```python
from build123d import *

# Parameters (mm, degrees)
SKETCH1_W               = 266.7
SKETCH1_H               = 215.9
BASE_FLANGE1_DEPTH      = 1.5748
SKETCH6_R               = 3.96875
CUT_EXTRUDE1_DEPTH      = 1.5748
SKETCH7_R               = 3.96875
CUT_EXTRUDE2_DEPTH      = 172.574779601
MIRROR2_COPY_1_SKETCH_R = 3.96875
MIRROR2_COPY_1_DEPTH    = 1.5748
MIRROR2_COPY_2_SKETCH_R = 3.96875
MIRROR2_COPY_2_DEPTH    = 172.574779601
SKETCH8_R               = 2.54
CUT_EXTRUDE3_DEPTH      = 172.574779601
SKETCH9_R               = 2.38125
CUT_EXTRUDE4_DEPTH      = 172.574779601


# Sheet-metal steps are written as plain solids
with BuildPart() as part:
    # Sketch1 → Base-Flange1 (new body)
    with BuildSketch(Plane(origin=(0, 0, 0), x_dir=(1, 0, 0), z_dir=(0, 1, 0))):
        Rectangle(SKETCH1_W, SKETCH1_H)
    extrude(amount=-BASE_FLANGE1_DEPTH)

    # Sketch6 → Cut-Extrude1 (cut)
    with BuildSketch(Plane(origin=(0, 0, 0), x_dir=(1, 0, 0), z_dir=(0, 1, 0))):
        with Locations(Location((-123.825, -82.55, 0), (0, 0, 270))):
            Circle(SKETCH6_R)
    cut_extrude1 = extrude(amount=-CUT_EXTRUDE1_DEPTH, mode=Mode.SUBTRACT)

    # Sketch7 → Cut-Extrude2 (cut, through all)
    with BuildSketch(Plane(origin=(0, 0, 0), x_dir=(1, 0, 0), z_dir=(0, 1, 0))):
        with Locations(Location((-63.5, -90.678, 0), (0, 0, 270))):
            Circle(SKETCH7_R)
    cut_extrude2 = extrude(amount=-CUT_EXTRUDE2_DEPTH, mode=Mode.SUBTRACT)

    # Mirror1: Cut-Extrude1, Cut-Extrude2 across plane
    add(cut_extrude1.mirror(Plane(origin=(0, 0, 0), x_dir=(0, 0, 1), z_dir=(1, 0, 0))), mode=Mode.SUBTRACT)
    add(cut_extrude2.mirror(Plane(origin=(0, 0, 0), x_dir=(0, 0, 1), z_dir=(1, 0, 0))), mode=Mode.SUBTRACT)

    # Mirror2: Cut-Extrude1, Cut-Extrude2 across plane
    add(cut_extrude1.mirror(Plane.XY), mode=Mode.SUBTRACT)
    add(cut_extrude2.mirror(Plane.XY), mode=Mode.SUBTRACT)

    # Mirror2 copy 1 sketch → Mirror2 copy 1 (cut)
    with BuildSketch(Plane(origin=(0, 0, 0), x_dir=(-1, 0, 0), z_dir=(0, 1, 0))):
        with Locations(Location((-123.825, -82.55, 0), (0, 0, 270))):
            Circle(MIRROR2_COPY_1_SKETCH_R)
    extrude(amount=-MIRROR2_COPY_1_DEPTH, mode=Mode.SUBTRACT)

    # Mirror2 copy 2 sketch → Mirror2 copy 2 (cut, through all)
    with BuildSketch(Plane(origin=(0, 0, 0), x_dir=(-1, 0, 0), z_dir=(0, 1, 0))):
        with Locations(Location((-63.5, -90.678, 0), (0, 0, 270))):
            Circle(MIRROR2_COPY_2_SKETCH_R)
    extrude(amount=-MIRROR2_COPY_2_DEPTH, mode=Mode.SUBTRACT)

    # Sketch8 → Cut-Extrude3 (cut, through all)
    with BuildSketch(Plane(origin=(0, 0, 0), x_dir=(1, 0, 0), z_dir=(0, 1, 0))):
        with Locations(Location((-82.55, -76.2, 0), (0, 0, 270))):
            Circle(SKETCH8_R)
        with Locations(Location((-31.75, -76.2, 0), (0, 0, 270))):
            Circle(SKETCH8_R)
        with Locations(Location((-82.55, 45.339, 0), (0, 0, 270))):
            Circle(SKETCH8_R)
        with Locations(Location((-31.75, 45.339, 0), (0, 0, 270))):
            Circle(SKETCH8_R)
    extrude(amount=-CUT_EXTRUDE3_DEPTH, mode=Mode.SUBTRACT)

    # Sketch9 → Cut-Extrude4 (cut, through all)
    with BuildSketch(Plane(origin=(0, 0, 0), x_dir=(1, 0, 0), z_dir=(0, 1, 0))):
        with Locations(Location((99.35, -81.95, 0), (0, 0, 270))):
            Circle(SKETCH9_R)
        with Locations(Location((16.35, 70.95, 0), (0, 0, 270))):
            Circle(SKETCH9_R)
    extrude(amount=-CUT_EXTRUDE4_DEPTH, mode=Mode.SUBTRACT)


solid = part.part
```
Can you work these out from the model? Positions are in its coordinate system, mm. Give positions to 0.01 mm unless a question says otherwise; leave off trailing zeros. Loops run counter-clockwise (first coordinate to the right, second up) from the corner with the lowest first, then second, coordinate; pieces in that order, holes last. Notation, with made-up numbers: M 61,49.25 L 95,49.25 A14 cw 95,70.25 Z; hole C 54.25,-33.5 d3. An arc over 180 degrees is marked long. One line per question, with ' | ' between items. Start each with the question number.
Q1. If we mould it in two halves opening along Z, with no side actions, what happens to faces 1 (the flat face through (-2, 0, -2)), 2 (the cylindrical face through (121.143, -0.776, 79.625))? For each: +Z half, -Z half, draft (parallel to the pull), parting line (faces both ways), or undercut.
Q2. If we section it at B-B (z = -82.55): Please give me the cut outline in (x, y), plus the area to 3 significant figures.
Q3. If we section it at A-A (x = 63.5): Please give me the cut outline in (y, z).
Q4. If I drill on line 1 (X direction, y = -0.5, z = 76.2); line 2 (Z direction, x = 61.5, y = -0.5); line 3 (X direction, y = -0.25, z = 83), over which ranges is the centre line in solid material (lowest first)? Write a range as from..to.
Q5. For pin 1 Ø6 at (x, z) = (-82.55, 76.2) entering from +Y, with a flat end and sliding along its axis, tell me the tip position at first contact or that it passes through.
Computed:
1) face 1: draft | face 2: undercut
2) outline: M -133.35,-1.57 L -127.79,-1.57 L -127.79,0 L -133.35,0 Z; M -119.86,-1.57 L 119.86,-1.57 L 119.86,0 L -119.86,0 Z; M 127.79,-1.57 L 133.35,-1.57 L 133.35,0 L 127.79,0 Z | area: 395 mm²
3) outline: M -1.57,-107.95 L 0,-107.95 L 0,-94.65 L -1.57,-94.65 Z; M -1.57,-86.71 L 0,-86.71 L 0,86.71 L -1.57,86.71 Z; M -1.57,94.65 L 0,94.65 L 0,107.95 L -1.57,107.95 Z
4) line 1: x = -133.35..-85.09, -80.01..-34.29, -29.21..133.35 | line 2: z = -107.95..-94.11, -87.25..87.25, 94.11..107.95 | line 3: x = -133.35..-127.77, -119.88..97.21, 101.49..119.88, 127.77..133.35
5) pin 1: stops at y = 0
